Geometry: final body of the model. Coordinates: model frame, mm. A direction names the side the tool comes from. Round coordinates to 2 decimals unless told otherwise and drop trailing zeros. Write each loop counter-clockwise with the first axis right and the second up, starting at its lowest first coordinate (ties: lowest second). Pieces come first, ordered by that corner, then holes. Notation, with made-up numbers: (57.5, 17.25) -> (63.5, 17.25) arc R29 ccw to (63.5, 45.25) -> close; hole circle Ø8 at (88, 29). An arc over 180 degrees is marked (long way). Use one line per item in the form item = value. Start each with the question number.
1. Draft query along Y for faces 4 (the face through (0, 31.75, 1)), 5 (the face through (0, 16, -38.1)), 6 (the face through (0, 0, 1)), 7 (the face through (15.668, 26.974, 3.664)). Return one class per face: pulls with the +Y half, pulls with the -Y half, needs draft (parallel to the pull), parting line crosses it, or undercut.
2. Cut plane A-A, the plane y = 22. State how many separate pieces and enclosed holes the cut face has, plus the area to 3 significant figures.
3. Cut plane B-B, the plane x = -5.5. Return the cut outline in (y, z), plus the area to 3 significant figures.
4. Cut plane D-D, the plane x = -11. Return the cut outline in (y, z), plus the area to 3 significant figures.
5. Pin query (flat end, axial travel): pin 1 Ø5 at (x, y) = (15.875, 25.4) entering from +Z; pin 2 Ø12.5 at (x, z) = (-0.5, -17) entering from -Y; pin 3 Ø1.9 at (x, z) = (15.875, -31.75) entering from +Y. Return the tip coordinate at first contact, or that it passes through.
6. Line query: L1, parallel to Z at x = 0, y = 8; L2, parallel to X at y = 26.5, z = -2.5; L3, parallel to Z at x = 10, y = 8. Output: solid intervals per line, ascending.
7. Reachability of faces 1 (the face through (19.05, 16, -1)), 2 (the face through (0, 25.4, -19)), 3 (the face through (-15.668, 23.826, 3.664)) from +Z, -Z, +X, -X, +Y, -Y: full face, straight path, thin tool, end or side. Return the list, or none.
```python
from build123d import *

# Parameters (mm, degrees)
F0_R     = 1.5875
F1_DEPTH = 31.75
F2_DEPTH = 25.4
F3_R     = 1.5875
F3_R_2   = 0.79375
F4_DEPTH = 69.85
F5_DEPTH = 69.85


with BuildPart() as f1:
    # F0 (on Front) → F1 (new body)
    with BuildSketch(Plane.XZ):
        with BuildLine():
            ThreePointArc((-14.2875, -31.75), (-15.875, -30.1625), (-17.4625, -31.75))
            ThreePointArc((-17.4625, -31.75), (-15.875, -33.3375), (-14.2875, -31.75))
        make_face()
        with Locations((15.875, -31.75)):
            Circle(F0_R)
        Polygon((19.05, -31.75), (19.05, 38.1), (-19.05, 38.1), (-19.05, -31.75), (-19.05, -38.1), (0, -38.1), (19.05, -38.1), align=None)
        with BuildLine():
            ThreePointArc((-14.2875, -31.75), (-15.875, -33.3375), (-17.4625, -31.75))
            ThreePointArc((-17.4625, -31.75), (-15.875, -30.1625), (-14.2875, -31.75))
        make_face(mode=Mode.SUBTRACT)
        with Locations((15.875, -31.75)):
            Circle(F0_R, mode=Mode.SUBTRACT)
        with BuildLine():
            ThreePointArc((12.7, -19.05), (8.980256, -28.030256), (0, -31.75))
            ThreePointArc((0, -31.75), (-8.980256, -10.069744), (12.7, -19.05))
        make_face(mode=Mode.SUBTRACT)
        with BuildLine():
            ThreePointArc((12.7, -19.05), (-8.980256, -10.069744), (0, -31.75))
            ThreePointArc((0, -31.75), (8.980256, -28.030256), (12.7, -19.05))
        make_face()
    extrude(amount=-F1_DEPTH)

    # F0 (on Front) → F2 (cut)
    with BuildSketch(Plane.XZ):
        with BuildLine():
            ThreePointArc((12.7, -19.05), (-8.980256, -10.069744), (0, -31.75))
            ThreePointArc((0, -31.75), (8.980256, -28.030256), (12.7, -19.05))
        make_face()
    extrude(amount=-F2_DEPTH, mode=Mode.SUBTRACT)

    # F3 (on face) → F4 (cut)
    with BuildSketch(Plane.XY.offset(38.1)):
        with Locations((15.875, 25.4)):
            Circle(F3_R)
        with Locations((15.875, 25.4)):
            Circle(F3_R_2, mode=Mode.SUBTRACT)
        with Locations((15.875, 25.4)):
            Circle(F3_R_2)
        with BuildLine():
            ThreePointArc((-14.2875, 25.4), (-15.875, 26.9875), (-17.4625, 25.4))
            ThreePointArc((-17.4625, 25.4), (-15.875, 23.8125), (-14.2875, 25.4))
        make_face()
        with BuildLine():
            ThreePointArc((-15.08125, 25.4), (-15.875, 24.60625), (-16.66875, 25.4))
            ThreePointArc((-16.66875, 25.4), (-15.875, 26.19375), (-15.08125, 25.4))
        make_face(mode=Mode.SUBTRACT)
        with BuildLine():
            ThreePointArc((-15.08125, 25.4), (-15.875, 26.19375), (-16.66875, 25.4))
            ThreePointArc((-16.66875, 25.4), (-15.875, 24.60625), (-15.08125, 25.4))
        make_face()
    extrude(amount=-F4_DEPTH, mode=Mode.SUBTRACT)

    # F3 (on face) → F5 (cut)
    with BuildSketch(Plane.XY.offset(38.1)):
        with BuildLine():
            ThreePointArc((-15.08125, 25.4), (-15.875, 26.19375), (-16.66875, 25.4))
            ThreePointArc((-16.66875, 25.4), (-15.875, 24.60625), (-15.08125, 25.4))
        make_face()
        with Locations((15.875, 25.4)):
            Circle(F3_R_2)
    extrude(amount=-F5_DEPTH, mode=Mode.SUBTRACT)


solid = f1.part
```
Outcome:
q1.face_4 = pulls with the +Y half
q1.face_5 = needs draft
q1.face_6 = pulls with the -Y half
q1.face_7 = undercut
q2.separate_pieces = 1
q2.enclosed_holes = 3
q2.area = 2,380 mm^2
q3.outline = (0, -38.1) -> (31.75, -38.1) -> (31.75, 38.1) -> (0, 38.1) -> (0, -7.6) -> (25.4, -7.6) -> (25.4, -30.5) -> (0, -30.5) -> close
q3.area = 1,840 mm^2
q4.outline = (0, -38.1) -> (31.75, -38.1) -> (31.75, 38.1) -> (0, 38.1) -> (0, -12.7) -> (25.4, -12.7) -> (25.4, -25.4) -> (0, -25.4) -> close
q4.area = 2,100 mm^2
q5.pin_1 = 38.1
q5.pin_2 = 25.4
q5.pin_3 = through
q6.L1 = -38.1 to -31.75, -6.35 to 38.1
q6.L2 = -19.05 to -17.02, -14.73 to 14.73, 17.02 to 19.05
q6.L3 = -38.1 to -26.88, -11.22 to 38.1
q7.face_1 = +Z, -Z, +X, +Y, -Y
q7.face_2 = -Y
q7.face_3 = +Z
